Could you check a few things on this model? Use its own coordinates, in mm. A direction names the side the tool comes from. Give positions to 0.01 mm unless a question says otherwise; leave off trailing zeros. Order: outer loops, then holes, each group sorted by start corner. A loop starts at its lowest first (then second) coordinate and runs counter-clockwise, first axis right, second up. Notation, with made-up numbers: (-34.75, 19) - (-12.75, 19) arc R16 cw to (-12.75, 44) - close; hole circle Ø8 at (59.25, 82). An arc over 180 degrees is marked (long way). One line per question, with ' | ' between items. Start each with the question number.
1. Imagine slicing it at C-C (z = -0.85). Give the number of separate pieces and of enclosed holes in the cut face, and give its area (3 significant figures).
2. Imagine slicing it at B-B (x = 58). Please give me the cut outline in (y, z), and give its area (3 significant figures).
3. Which directions (+Z, -Z, +X, -X, +Y, -Y) give clear straight access to the entire face, cutting with the end or side of a thin tool? Please do faces 1 (the flat face through (-90, 124, 0)), 2 (the flat face through (-70, -176, 0)), 3 (the flat face through (138.6, 170.9, 0)).
4. I need wall thicknesses on probe 1 along Y at (x, z) = (-109.5, -0.05); probe 2 along X at (y, z) = (-150, 0.5); probe 3 along X at (y, z) = (-90, 0.9). Which ranges of each line are inside material? Lowest first, please. Write a range as from..to.
5. If we mould it in two halves opening along X, with no side actions, what happens to faces 4 (the flat face through (-90, -123, 0)), 5 (the flat face through (-101, 3, 2)), 6 (the flat face through (-138.6, 170.9, 0))? For each: released by +X, released by -X, zero draft, split by the parting line, or undercut.
6. For P1, Ø1.2, axis at x = -10, z = 1, coming from the -Y side, with a flat end and sliding along its axis, tell me the tip position at first contact or that it passes through.
7. Imagine slicing it at A-A (y = 36.5). Please give me the cut outline in (x, z).
Autodesk Inventor part; units mm, degrees
ref_plane "YZ Plane" through (0, 0, 0) normal (1, 0, 0) x (0, 1, 0)
ref_plane "XZ Plane" through (0, 0, 0) normal (0, 1, 0) x (-1, 0, 0)
ref_plane "XY Plane" through (0, 0, 0) normal (0, 0, 1) x (1, 0, 0)
sketch "Hinges" plane through (0, 0, 0) normal (0, 0, 1) x (1, 0, 0)
  circle A0 centre (-464.8647, 95.9101) radius 1.75
  circle A1 centre (-464.8647, 121.4101) radius 1.75
  line L0 (-471.3647, 88.6601) -> (-455.3647, 88.6601)
  line L1 (-455.3647, 88.6601) -> (-455.3647, 128.6601)
  line L2 (-455.3647, 128.6601) -> (-471.3647, 128.6601)
  line L3 (-471.3647, 128.6601) -> (-471.3647, 88.6601)
  circle A2 centre (-439.8647, 121.4101) radius 1.75
  circle A3 centre (-439.8647, 95.9101) radius 1.75
  line L4 (-433.3647, 128.6601) -> (-449.3647, 128.6601)
  line L5 (-449.3647, 128.6601) -> (-449.3647, 88.6601)
  line L6 (-449.3647, 88.6601) -> (-433.3647, 88.6601)
  line L7 (-433.3647, 88.6601) -> (-433.3647, 128.6601)
  point P0 (-452.3647, 108.6601)
  dimension "d30" = 3.5
  dimension "d31" = 25.5
  dimension "d32" = 6.5
  dimension "d33" = 40
  dimension "d34" = 7.25
  dimension "d35" = 16
  dimension "d36" = 3.5
  dimension "d37" = 25.5
  dimension "d38" = 6.5
  dimension "d39" = 40
  dimension "d40" = 7.25
  dimension "d41" = 16
  dimension "d42" = 38
sketch "Sketch1" plane through (0, 0, 0) normal (0, 0, 1) x (1, 0, 0)
  line L0 (-148.5, 181) -> (148.5, 181)
  line L1 (148.5, 181) -> (148.5, -181)
  line L2 (148.5, -181) -> (-148.5, -181)
  line L3 (-148.5, -181) -> (-148.5, 181)
  line L4 (-75, -181) -> (-65, -171)
  line L5 (-75, -181) -> (-60.8579, -181) construction
  line L6 (-65, -171) -> (65, -171)
  line L7 (65, -171) -> (75, -181)
  line L8 (-125, -181) -> (-148.5, -157.5)
  line L9 (-125, -181) -> (-91.766, -181) construction
  line L10 (125, -181) -> (148.5, -157.5)
  line L11 (125, -181) -> (158.234, -181) construction
  line L12 (-148.5, 161) -> (-128.5, 181)
  line L13 (-148.5, 161) -> (-120.2157, 161) construction
  line L14 (148.5, 161) -> (128.5, 181)
  line L15 (-100, 134) -> (100, 134)
  line L16 (100, 134) -> (100, -133)
  line L17 (100, -133) -> (-100, -133)
  line L18 (-100, -133) -> (-100, 134)
  point P0 (0, 0)
  point P1 (0, 181)
  point P2 (-148.5, 0)
  point P3 (0, -171)
  point P4 (0, 134)
  dimension "d0" = 297
  dimension "d1" = 362
  dimension "d2" = 45
  dimension "d3" = 10
  dimension "d4" = 150
  dimension "d5" = 135
  dimension "d6" = 50
  dimension "d7" = 45
  dimension "d8" = 50
  dimension "d9" = 45
  dimension "d10" = 20
  dimension "d11" = 20
  dimension "d12" = 135
  dimension "d13" = 47
  dimension "d14" = 200
  dimension "d15" = 267
extrude "Extrusion1" add sketch "Sketch1" along normal mid plane 4 contours L0 L14 L1 L10 L2 L7 L6 L4 L8 L3 L12
chamfer "Chamfer1" distance 20 angle 45 4 edges at (-100, 134, 0) (100, 134, 0) (-100, -133, 0) (100, -133, 0)
sketch "Sketch3" plane through (0, 0, -2) normal (0, 0, -1) x (-1, 0, 0)
  circle A0 centre (-140.5, 150) radius 3
  circle A1 centre (-140.5, -150) radius 3
  circle A2 centre (140.5, -150) radius 3
  circle A3 centre (140.5, 150) radius 3
  line L0 (-148.5, 161) -> (-148.5, -157.5)
  line L1 (148.5, -157.5) -> (148.5, 161)
  point P0 (0, 0)
  dimension "d25" = 6
  dimension "d26" = 300
  dimension "d27" = 150
  dimension "d47" = 8
  dimension "d48" = 8
extrude "Extrusion3" cut sketch "Sketch3" against normal blind 37.5
sketch "Sketch4" plane through (0, 0, -2) normal (0, 0, -1) x (-1, 0, 0)
  line L0 (100, 114) -> (100, -113)
  line L1 (-100, -113) -> (-100, 114)
  circle A0 centre (84.5, 71.25) radius 1.75
  circle A1 centre (84.5, 96.75) radius 1.75
  line L2 (78, 64) -> (94, 64)
  line L3 (94, 64) -> (94, 104)
  line L4 (94, 104) -> (78, 104)
  line L5 (78, 104) -> (78, 64)
  circle A2 centre (109.5, 96.75) radius 1.75
  circle A3 centre (109.5, 71.25) radius 1.75
  line L6 (116, 104) -> (100, 104)
  line L7 (100, 104) -> (100, 64)
  line L8 (100, 64) -> (116, 64)
  line L9 (116, 64) -> (116, 104)
  circle A4 centre (84.5, -95.75) radius 1.75
  circle A5 centre (84.5, -70.25) radius 1.75
  line L10 (78, -103) -> (94, -103)
  line L11 (94, -103) -> (94, -63)
  line L12 (94, -63) -> (78, -63)
  line L13 (78, -63) -> (78, -103)
  circle A6 centre (109.5, -70.25) radius 1.75
  circle A7 centre (109.5, -95.75) radius 1.75
  line L14 (116, -63) -> (100, -63)
  line L15 (100, -63) -> (100, -103)
  line L16 (100, -103) -> (116, -103)
  line L17 (116, -103) -> (116, -63)
  circle A8 centre (-109.5, -12.75) radius 1.75
  circle A9 centre (-109.5, 12.75) radius 1.75
  line L18 (-116, -20) -> (-100, -20)
  line L19 (-100, -20) -> (-100, 20)
  line L20 (-100, 20) -> (-116, 20)
  line L21 (-116, 20) -> (-116, -20)
  circle A10 centre (-84.5, 12.75) radius 1.75
  circle A11 centre (-84.5, -12.75) radius 1.75
  line L22 (-78, 20) -> (-94, 20)
  line L23 (-94, 20) -> (-94, -20)
  line L24 (-94, -20) -> (-78, -20)
  line L25 (-78, -20) -> (-78, 20)
  point P0 (0, 0)
  point P1 (-100, 0)
  dimension "d43" = 10
  dimension "d44" = 10
extrude "Extrusion4" cut sketch "Sketch4" against normal blind 10 contours A2 | A3 | A6 | A7 | A8 | A9
equation "\"d34\" = -0.5 * d31 + 0.5 * d33"
equation "\"d40\" = -0.5 * d37 + 0.5 * d39"
equation "\"d8\" = d6"
equation "\"d48\" = d47"
properties part number "Sides Covers" material "Wood (Birch)"
Results found:
1) separate pieces: 1 | enclosed holes: 11 | area: 52,400 mm2
2) outline: (-171, -2) - (-133, -2) - (-133, 2) - (-171, 2) - close; (134, -2) - (181, -2) - (181, 2) - (134, 2) - close | area: 340 mm2
3) face 1: +Z, -Z | face 2: +Z, -Z, -Y | face 3: +Z, -Z, +X, +Y
4) probe 1: y = -181..-97.5, -94..-72, -68.5..69.5, 73..95, 98.5..181 | probe 2: x = -148.5..-143.5, -137.5..137.5, 143.5..148.5 | probe 3: x = -148.5..-100, 100..148.5
5) face 4: undercut | face 5: zero draft | face 6: released by -X
6) P1: stops at y = -171
7) outline: (-148.5, -2) - (-100, -2) - (-100, 2) - (-148.5, 2) - close; (100, -2) - (148.5, -2) - (148.5, 2) - (100, 2) - close
